CAD build for the part. Positions are in the model's coordinates, mm. A direction names the side the tool comes from. Coordinates: 2 decimals unless noted, no trailing zeros. Loops run counter-clockwise (first coordinate to the right, second up) from the corner with the lowest first, then second, coordinate; pieces in that order, holes last. Notation, with made-up numbers: (-26, 89.5) -> (21, 89.5) arc R18 ccw to (21, 101.5) -> close; hole circle Ø5 at (-7, 64). An arc over 180 degrees is marked (long way). Write item = value, one per line. Start each with the question number.
(1) Drill centre lines: line 1 (X direction, y = -2, z = -20.5); line 2 (Z direction, x = 22.75, y = 0). Where is each one in solid material? Low to high. Write a range as from..to.
(2) Band-saw the part on B-B (z = 0). Write the cut outline in (x, y).
(3) Band-saw the part on D-D (x = 34). Write the cut outline in (y, z).
(4) Pull direction X, two halves, no side cores. Call faces 6 (the face through (15, 1.4, 18.1)), 7 (the face through (0, 0, 0)), 8 (the face through (10, 0, -25)), 9 (the face through (9.944, -2.799, -21.317)): +X half, -X half, draft (parallel to the pull), parting line (faces both ways), or undercut.
(5) Band-saw the part on C-C (y = 0). Write the cut outline in (x, z).
(6) Tool access for faces 1 (the face through (45, -10.3, 18.2)), 2 (the face through (20, 0, -26)), 3 (the face through (10, 0, 25)), 4 (the face through (28.557, -2.343, -17.847)), 5 (the face through (5, 0, 0)): list every direction of +Z, -Z, +X, -X, +Y, -Y with a clear straight run to the whole face (end or side of a thin tool).
(7) Band-saw the part on A-A (x = 9.5). Write the cut outline in (y, z), and give its area (3 significant figures).
(8) Flat gauge pins, fed straight in: P1, Ø4, axis at x = 14, z = 6.5, coming from the +Y side; P2, Ø1, axis at x = 24, y = 5.5, coming from the -Z side; P3, Ø20.5, axis at y = -5.5, z = 1, coming from the +X side; P4, Ø4, axis at y = 9, z = 1, coming from the -X side. Where does each tip first touch, or does it go through?
Autodesk Inventor part; units mm, degrees
ref_plane "YZ Plane" through (0, 0, 0) normal (1, 0, 0) x (0, 1, 0)
ref_plane "XZ Plane" through (0, 0, 0) normal (0, 1, 0) x (-1, 0, 0)
ref_plane "XY Plane" through (0, 0, 0) normal (0, 0, 1) x (1, 0, 0)
sketch "Esboço1" plane through (0, 0, 0) normal (0, 0, 1) x (1, 0, 0)
  line L0 (0, 0) -> (0, 27.5)
  line L1 (0, 27.5) -> (45, 27.5)
  line L2 (45, 27.5) -> (45, 18)
  line L3 (45, 18) -> (15, 18)
  line L4 (15, 18) -> (15, 20.5)
  line L5 (14, 21.5) -> (6, 21.5)
  line L6 (5, 20.5) -> (5, 0)
  line L7 (5, 0) -> (0, 0)
  arc A0 (6, 21.5) -> (5, 20.5) centre (6, 20.5) ccw
  arc A1 (15, 20.5) -> (14, 21.5) centre (14, 20.5) ccw
  point P0 (15, 21.5)
  point P1 (5, 21.5)
  point P2 (2.5, 0)
  dimension "d0" = 55
  dimension "d1" = 45
  dimension "d2" = 40
  dimension "d3" = 10
  dimension "d4" = 43
  dimension "d5" = 36
  dimension "d7" = 1
revolve "Revolução1" add sketch "Esboço1" angle 360 about axis through (5, 0, 0) along (-1, 0, 0)
thread "Rosca1"
chamfer "Chanfro1" distance 2.5 angle 45 1 edges at (45, -18, 0)
chamfer "Chanfro2" distance 2 angle 45 1 edges at (0, -27.5, 0)
sketch "Esboço2" plane through (0, 0, 0) normal (-1, 0, 0) x (0, 0, 1)
  line L0 (35, 15) -> (25, 15)
  line L1 (25, 15) -> (25, -15)
  line L2 (25, -15) -> (35, -15)
  line L3 (35, -15) -> (35, 15)
  line L4 (0, 0) -> (0, 48.3758) construction
  line L5 (-35, 15) -> (-25, 15)
  line L6 (-25, 15) -> (-25, -15)
  line L7 (-25, -15) -> (-35, -15)
  line L8 (-35, -15) -> (-35, 15)
  point P0 (25, 0)
  point P1 (35, 0)
  point P2 (30, -15)
  point P3 (-25, 0)
  point P4 (-35, 0)
  point P5 (-30, -15)
  dimension "d17" = 25
  dimension "d18" = 30
  dimension "d19" = 10
extrude "Extrusão1" cut sketch "Esboço2" against normal blind 20
properties part number "3D Model"
Findings below:
q1.line_1 = 0..5, 15..45
q1.line_2 = -27.5..-18, 18..27.5
q2.outline = (0, -25.5) -> (2, -27.5) -> (45, -27.5) -> (45, -20.5) -> (42.5, -18) -> (15, -18) -> (15, -20.5) arc R1 cw to (14, -21.5) -> (6, -21.5) arc R1 cw to (5, -20.5) -> (5, 20.5) arc R1 cw to (6, 21.5) -> (14, 21.5) arc R1 cw to (15, 20.5) -> (15, 18) -> (42.5, 18) -> (45, 20.5) -> (45, 27.5) -> (2, 27.5) -> (0, 25.5) -> close
q3.outline = circle Ø55 at (0, 0); hole circle Ø36 at (0, 0)
q4.face_6 = undercut
q4.face_7 = -X half
q4.face_8 = draft
q4.face_9 = undercut
q5.outline = (0, -25) -> (20, -25) -> (20, -27.5) -> (45, -27.5) -> (45, -20.5) -> (42.5, -18) -> (15, -18) -> (15, -20.5) arc R1 cw to (14, -21.5) -> (6, -21.5) arc R1 cw to (5, -20.5) -> (5, 20.5) arc R1 cw to (6, 21.5) -> (14, 21.5) arc R1 cw to (15, 20.5) -> (15, 18) -> (42.5, 18) -> (45, 20.5) -> (45, 27.5) -> (20, 27.5) -> (20, 25) -> (0, 25) -> close
q6.face_1 = +Z, -Z, +X, +Y, -Y
q6.face_2 = -Z, -X, +Y, -Y
q6.face_3 = +Z, -X, +Y, -Y
q6.face_4 = +X
q6.face_5 = none
q7.outline = (-11.46, -25) -> (11.46, -25) arc R27.5 ccw to (11.46, 25) -> (-11.46, 25) arc R27.5 ccw to start; hole circle Ø43 at (0, 0)
q7.area = 847 mm²
q8.P1 = 27.13
q8.P2 = -27.04
q8.P3 = 5
q8.P4 = 0
